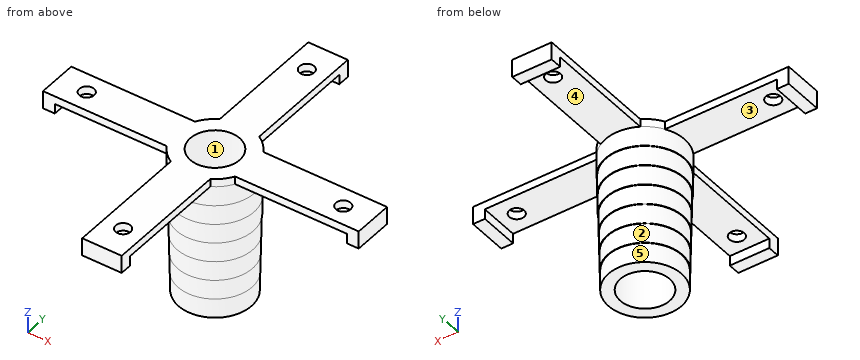
from build123d import *

# Parameters (mm, degrees)
SKETCH1_R               = 10
BOSS_EXTRUDE1_DEPTH     = 5
SKETCH2_W               = 5
SKETCH2_H               = 5
BOSS_EXTRUDE2_DEPTH     = 2
SKETCH3_R               = 9.875
BOSS_EXTRUDE3_DEPTH     = 5
SKETCH4_R               = 9.75
BOSS_EXTRUDE4_DEPTH     = 5
SKETCH5_R               = 9.625
BOSS_EXTRUDE5_DEPTH     = 5
SKETCH6_R               = 9.5
BOSS_EXTRUDE6_DEPTH     = 5
SKETCH7_R               = 9.375
BOSS_EXTRUDE7_DEPTH     = 5
SKETCH8_R               = 9.25
BOSS_EXTRUDE8_DEPTH     = 5
SKETCH9_W               = 3
SKETCH9_H               = 10
SKETCH9_W_2             = 10
SKETCH9_H_2             = 3
BOSS_EXTRUDE9_DEPTH     = 2.5
CUT_EXTRUDE1_DEPTH      = 67.520673478
CUT_EXTRUDE1_DEPTH_BACK = 67.520673478
SKETCH10_R              = 1.875
CUT_EXTRUDE2_DEPTH      = 68.594378464
CUT_EXTRUDE2_DEPTH_BACK = 68.594378464
SKETCH11_R              = 6.25


with BuildPart() as part:
    # Sketch1 → Boss-Extrude1 (new body)
    with BuildSketch(Plane.XY):
        Circle(SKETCH1_R)
    extrude(amount=BOSS_EXTRUDE1_DEPTH)

    # Sketch2 → Boss-Extrude2 (add)
    with BuildSketch(Plane.XY.offset(5)):
        with BuildLine():
            ThreePointArc((-8.660254038, -5), (-10, 0), (-8.660254038, 5))
            Line((-8.660254038, 5), (-40, 5))
            Line((-40, 5), (-40, -5))
            Line((-40, -5), (-8.660254038, -5))
        make_face()
        with BuildLine():
            Line((-5, 0), (-5, 5))
            Line((-5, 5), (-8.660254038, 5))
            ThreePointArc((-8.660254038, 5), (-10, 0), (-8.660254038, -5))
            Line((-8.660254038, -5), (-5, -5))
            Line((-5, -5), (-5, 0))
        make_face()
        with BuildLine():
            Line((-5, 40), (-5, 8.660254038))
            ThreePointArc((-5, 8.660254038), (0, 10), (5, 8.660254038))
            Line((5, 8.660254038), (5, 40))
            Line((5, 40), (-5, 40))
        make_face()
        with BuildLine():
            Line((-5, 5), (0, 5))
            Line((0, 5), (5, 5))
            Line((5, 5), (5, 8.660254038))
            ThreePointArc((5, 8.660254038), (0, 10), (-5, 8.660254038))
            Line((-5, 8.660254038), (-5, 5))
        make_face()
        with BuildLine():
            Line((40, 5), (8.660254038, 5))
            ThreePointArc((8.660254038, 5), (9.659258263, 2.588190451), (10, 0))
            ThreePointArc((10, 0), (9.659258263, -2.588190451), (8.660254038, -5))
            Line((8.660254038, -5), (40, -5))
            Line((40, -5), (40, 5))
        make_face()
        with BuildLine():
            Line((8.660254038, 5), (5, 5))
            Line((5, 5), (5, 0))
            Line((5, 0), (5, -5))
            Line((5, -5), (8.660254038, -5))
            ThreePointArc((8.660254038, -5), (9.659258263, -2.588190451), (10, 0))
            ThreePointArc((10, 0), (9.659258263, 2.588190451), (8.660254038, 5))
        make_face()
        with BuildLine():
            ThreePointArc((5, -8.660254038), (0, -10), (-5, -8.660254038))
            Line((-5, -8.660254038), (-5, -40))
            Line((-5, -40), (5, -40))
            Line((5, -40), (5, -8.660254038))
        make_face()
        with BuildLine():
            Line((5, -5), (0, -5))
            Line((0, -5), (-5, -5))
            Line((-5, -5), (-5, -8.660254038))
            ThreePointArc((-5, -8.660254038), (0, -10), (5, -8.660254038))
            Line((5, -8.660254038), (5, -5))
        make_face()
        with Locations((2.5, -2.5)):
            Rectangle(SKETCH2_W, SKETCH2_H)
        with Locations((-2.5, -2.5)):
            Rectangle(SKETCH2_W, SKETCH2_H)
        with Locations((2.5, 2.5)):
            Rectangle(SKETCH2_W, SKETCH2_H)
        with Locations((-2.5, 2.5)):
            Rectangle(SKETCH2_W, SKETCH2_H)
        with BuildLine():
            Line((-8.660254038, 5), (-5, 5))
            Line((-5, 5), (-5, 8.660254038))
            ThreePointArc((-5, 8.660254038), (-7.071067812, 7.071067812), (-8.660254038, 5))
        make_face()
        with BuildLine():
            Line((5, 8.660254038), (5, 5))
            Line((5, 5), (8.660254038, 5))
            ThreePointArc((8.660254038, 5), (7.071067812, 7.071067812), (5, 8.660254038))
        make_face()
        with BuildLine():
            Line((8.660254038, -5), (5, -5))
            Line((5, -5), (5, -8.660254038))
            ThreePointArc((5, -8.660254038), (7.071067812, -7.071067812), (8.660254038, -5))
        make_face()
        with BuildLine():
            Line((-5, -5), (-8.660254038, -5))
            ThreePointArc((-8.660254038, -5), (-7.071067812, -7.071067812), (-5, -8.660254038))
            Line((-5, -8.660254038), (-5, -5))
        make_face()
    extrude(amount=BOSS_EXTRUDE2_DEPTH)

    # Sketch3 → Boss-Extrude3 (add)
    with BuildSketch(Plane(origin=(0, 0, 0), x_dir=(-1, 0, 0), z_dir=(0, 0, -1))):
        Circle(SKETCH3_R)
    extrude(amount=BOSS_EXTRUDE3_DEPTH)

    # Sketch4 → Boss-Extrude4 (add)
    with BuildSketch(Plane(origin=(0, 0, -5), x_dir=(-1, 0, 0), z_dir=(0, 0, -1))):
        Circle(SKETCH4_R)
    extrude(amount=BOSS_EXTRUDE4_DEPTH)

    # Sketch5 → Boss-Extrude5 (add)
    with BuildSketch(Plane(origin=(0, 0, -10), x_dir=(-1, 0, 0), z_dir=(0, 0, -1))):
        Circle(SKETCH5_R)
    extrude(amount=BOSS_EXTRUDE5_DEPTH)

    # Sketch6 → Boss-Extrude6 (add)
    with BuildSketch(Plane(origin=(0, 0, -15), x_dir=(-1, 0, 0), z_dir=(0, 0, -1))):
        Circle(SKETCH6_R)
    extrude(amount=BOSS_EXTRUDE6_DEPTH)

    # Sketch7 → Boss-Extrude7 (add)
    with BuildSketch(Plane(origin=(0, 0, -20), x_dir=(-1, 0, 0), z_dir=(0, 0, -1))):
        Circle(SKETCH7_R)
    extrude(amount=BOSS_EXTRUDE7_DEPTH)

    # Sketch8 → Boss-Extrude8 (add)
    with BuildSketch(Plane(origin=(0, 0, -25), x_dir=(-1, 0, 0), z_dir=(0, 0, -1))):
        Circle(SKETCH8_R)
    extrude(amount=BOSS_EXTRUDE8_DEPTH)

    # Sketch9 → Boss-Extrude9 (add)
    with BuildSketch(Plane(origin=(0, 0, 5), x_dir=(-1, 0, 0), z_dir=(0, 0, -1))):
        with Locations((-38.5, 0)):
            Rectangle(SKETCH9_W, SKETCH9_H)
        with Locations((0, 38.5)):
            Rectangle(SKETCH9_W_2, SKETCH9_H_2)
        with Locations((38.5, 0)):
            Rectangle(SKETCH9_W, SKETCH9_H)
        with Locations((0, -38.5)):
            Rectangle(SKETCH9_W_2, SKETCH9_H_2)
    extrude(amount=BOSS_EXTRUDE9_DEPTH)

    # Sketch10 → Cut-Extrude1 (cut, two sides: drawn at the far end of the back side and taken through both)
    with BuildSketch(Plane(origin=(0, 0, 5), x_dir=(-1, 0, 0), z_dir=(0, 0, -1)).offset(-CUT_EXTRUDE1_DEPTH_BACK)):
        with Locations((-32.5, 0)):
            Circle(SKETCH10_R)
        with Locations((0, 32.5)):
            Circle(SKETCH10_R)
        with Locations((32.5, 0)):
            Circle(SKETCH10_R)
        with Locations((0, -32.5)):
            Circle(SKETCH10_R)
    extrude(amount=CUT_EXTRUDE1_DEPTH + CUT_EXTRUDE1_DEPTH_BACK, mode=Mode.SUBTRACT)

    # Sketch11 → Cut-Extrude2 (cut, two sides: drawn at the far end of the back side and taken through both)
    with BuildSketch(Plane(origin=(0, 0, -30), x_dir=(-1, 0, 0), z_dir=(0, 0, -1)).offset(-CUT_EXTRUDE2_DEPTH_BACK)):
        Circle(SKETCH11_R)
    extrude(amount=CUT_EXTRUDE2_DEPTH + CUT_EXTRUDE2_DEPTH_BACK, mode=Mode.SUBTRACT)


solid = part.part
Work out the finished part from the listing and answer in its coordinate system (mm). Face numbers are marked on the shaded views. A direction names the side the tool comes from. Round coordinates to 2 decimals unless told otherwise and drop trailing zeros. Order: outer loops, then holes, each group sorted by start corner. A loop starts at its lowest first (then second) coordinate and runs counter-clockwise, first axis right, second up. Notation, with made-up numbers: M 74.5,46 L 78.5,46 A21 ccw 78.5,61 Z; hole C -1.5,-32 d10. An arc over 180 degrees is marked long. Put each result on its own line as item: value. Start each with the question number.
Q1. For a pull along X with two mould halves and no side action, classify the marked faces 3, 4 and 5 as pulls with the +X half, pulls with the -X half, needs draft (parallel to the pull), parting line crosses it, or undercut.
Q2. A tool of negligible diameter and unlimited length cuts with its end or side. For the marked faces 1 and 2, from which of +Z, -Z, +X, -X, +Y, -Y can it reach the whole face along a straight path? Write none if from no direction.
Q3. Section A-A, the plane x = 32.5 is taken. Write down the section's boundary in (y, z) (3 decimals).
Q4. Section C-C, the plane x = 0 is taken. Give the number of separate pieces and of enclosed holes in the cut face, and give its area (3 significant figures).
Q5. Section B-B, the plane z = -3 is taken. Write down the section's boundary in (x, y) (3 decimals), and give its area (3 significant figures).
Q6. Section D-D, the plane y = 28.5 is taken. Write down the section's boundary in (x, z), and give its area (3 significant figures).
Q7. Flat-ended cylindrical pins translate along their axes: pin 1 (5 mm diameter, centred on y = -27, z = 5, fed in from +X); pin 2 (5 mm diameter, centred on x = 24, y = 2, fed in from -Z); pin 3 (6 mm diameter, centred on x = 1, y = 3, fed in from -Z); pin 4 (2 mm diameter, centred on x = 26, z = 5, fed in from -Y). Find the tip coordinate at first contact, or state that the pin passes through.
Q8. Straight lines are drawn through the part: L1, parallel to X at y = 0, z = 6.4 (3 decimals); L2, parallel to Y at x = -32.5, z = 5.8 (3 decimals). For each, find the intervals that lie inside material, in ascending order. Write a range as [from, to].
Findings below:
1. face 3: undercut
1. face 4: needs draft
1. face 5: parting line crosses it
2. face 1: +Z, -Z
2. face 2: -Z
3. outline: M -5,5 L -1.875,5 L -1.875,7 L -5,7 Z; M 1.875,5 L 5,5 L 5,7 L 1.875,7 Z
4. separate pieces: 4
4. enclosed holes: 0
4. area: 371 mm^2
5. outline: C 0,0 d19.75; hole C 0,0 d12.5
5. area: 184 mm^2
6. outline: M -5,5 L 5,5 L 5,7 L -5,7 Z
6. area: 20.0 mm^2
7. pin 1: stops at x = 5
7. pin 2: stops at z = 5
7. pin 3: passes through
7. pin 4: stops at y = -5
8. L1: x = [-40, -34.375], [-30.625, -6.25], [6.25, 30.625], [34.375, 40]
8. L2: y = [-5, -1.875], [1.875, 5]
